Autodesk Inventor part; units mm, degrees
ref_plane "Płaszczyzna konstrukcyjna4" through (813.3596, 0, 43.2274) normal (0.1218693, 0, -0.9925462) x (0, 1, 0)
ref_plane "YZ Plane" through (0, 0, 0) normal (1, 0, 0) x (0, 1, 0)
ref_plane "XZ Plane" through (0, 0, 0) normal (0, 1, 0) x (-1, 0, 0)
sketch "Szkic1" plane through (0, 0, 0) normal (1, 0, 0) x (0, 1, 0)
  circle A0 centre (0, 0) radius 16
  dimension "d0" = 32
extrude "Wyciągnięcie proste1" add sketch "Szkic1" along normal blind 815
shell "Skorupa1" thickness 2 removed faces 2 at (815, 4.7224, 2.4785) at (0, 4.7224, 2.4785)
sketch "Szkic4" plane through (0, 0, 0) normal (0, 0, 1) x (1, 0, 0)
  line L0 (320, 29.1092) -> (320, -35.5658)
  line L1 (0, 16) -> (0, -16)
  point P0 (0, 0)
  dimension "d8" = 320
bend part "Gięcie części1" radius 163.7022 angle 7 line through (320, 29.1092, 0) along (0, -1, 0) centre toward (0, 0, 1) moving side (1, 0, 0) both sides no
sketch "Szkic7" plane through (811.4097, 0, 59.1081) normal (0.9925462, 0, 0.1218693) x (0.1218693, 0, -0.9925462)
  circle A0 centre (0, 0) radius 14
  circle A1 centre (0, 0) radius 16
  point P0 (-40.2184, 0)
  point P1 (16, 0)
ref_plane "Płaszczyzna konstrukcyjna4" through (813.3596, 0, 43.2274) normal (0.1218693, 0, -0.9925462) x (0, 1, 0)
sketch "Szkic8" plane through (813.3596, 0, 43.2274) normal (0.1218693, 0, -0.9925462) x (0, 1, 0)
  line L0 (-19.5179, -302.5651) -> (38.9, -302.5651)
  ellipse E0 centre (0, -812.5651) end of major axis (-16, -812.5651) minor radius 1.9499
  dimension "d15" = 510
bend part "Gięcie części2" radius 35.4407 angle 97 line through (513.0498, -19.5179, 6.354) along (0, 1, 0) centre toward (0.1218693, 0, -0.9925462) moving side (0.9925462, 0, 0.1218693) both sides no
sketch "Szkic10" plane through (0, 0, 0) normal (0, 0, 1) x (1, 0, 0)
  line L0 (0, 16) -> (0, -16) construction
  line L1 (0, -16) -> (320, -16) construction
  line L2 (0, 16) -> (0, -16)
  line L3 (0, -16) -> (2.7996, -16)
  line L4 (2.7996, -16) -> (0, 16)
  point P0 (0, 0)
  dimension "d22" = 5
extrude "Wyciągnięcie proste4" cut sketch "Szkic10" along normal mid plane 32
equation "\"PromieńGięcia\" = Grubość"
equation "\"SzerokośćGięciaPodcięcia\" = Grubość"
equation "\"GłębokośćGięciaPodcięcia\" = 0.5 * Grubość"
equation "\"RozmiarPodcięciaNarożnika\" = 4 * Grubość"
equation "\"MinimalnaPozostałość\" = 2 * Grubość"
equation "\"PromieńPrzejścia\" = PromieńGięcia"
equation "\"Rozmiar_promienia_Jacobiego\" = Grubość"
equation "\"Wielk_odstępu\" = Grubość"
properties part number "Rura_podłużna_ergosiedziska_lewa" material "Aluminium AW-7020"
CAD build for the part. Positions are in the model's coordinates, mm. A direction names the side the tool comes from. Coordinates: 2 decimals unless noted, no trailing zeros. Write each loop counter-clockwise with the first axis right and the second up, starting at its lowest first coordinate (ties: lowest second). Pieces come first, ordered by that corner, then holes.
(1) Two-plate mould, pull along Y, no slides. Class faces 4 (the face through (554.7, 1.1, -271.388)), 5 (the face through (157.848, 12.932, 5.362)), 6 (the face through (423.58, 14.78, 17.66)): +Y half, -Y half, draft (parallel to the pull), parting line (faces both ways), or undercut.
(2) 3-axis set-ups, long thin cutter, end or side, ignore diameter. For faces 1 (the face through (157.76, -3.47, 15.62)), 2 (the face through (584.43, -3.47, -148.41)), 3 (the face through (424.84, 13.354, 7.406)): which of +Z, -Z, +X, -X, +Y, -Y reach the whole face in a straight line?
(3) Cut at A-A, the plane y = 0. List the corners of the cut face in (x, z), and give its area (3 significant figures).
(4) Flat gauge pins, fed straight in: pin 1 (12 mm diameter, centred on y = 1.5, z = -57, fed in from +X); pin 2 (6 mm diameter, centred on x = 242, y = 3, fed in from +Z); pin 3 (1.5 mm diameter, centred on x = 191, y = -3.5, fed in from +Z); pin 4 (10 mm diameter, centred on y = 12.5, z = -104, fed in from +X). Where does each tip first touch, or does it go through?
(5) Cut at B-B, the plane x = 118.5. List the corners of the cut face in (y, z).
(6) Cut at C-C, the plane z = -43. List the corners of the cut face in (x, y), and give its area (3 significant figures).
(7) Drill centre lines: probe 1 along Y at (x, z) = (213.5, 0); probe 2 along X at (y, z) = (0, -104). Where is each one in solid material? Low to high.
Geometry says:
1. face 4: draft
1. face 5: undercut
1. face 6: parting line
2. face 1: -X
2. face 2: -Z
2. face 3: none
3. outline: (1.4, -16) - (320, -16) arc R179.7 ccw to (341.9, -14.66) - (513.05, 6.35) arc R35.44 cw to (552.81, -28.82) - (552.81, -271.39) - (554.81, -271.39) - (554.81, -28.82) arc R37.44 ccw to (512.81, 8.34) - (341.66, -12.68) arc R177.7 cw to (320, -14) - (1.4, -14) - close; (1.4, 14) - (320, 14) arc R149.7 ccw to (338.24, 15.12) - (509.39, 36.13) arc R65.44 cw to (582.81, -28.82) - (582.81, -271.39) - (584.81, -271.39) - (584.81, -28.82) arc R67.44 ccw to (509.15, 38.12) - (338, 17.1) arc R147.7 cw to (320, 16) - (1.4, 16) - close
3. area: 3,360 mm2
4. pin 1: stops at x = 584.81
4. pin 2: stops at z = 16
4. pin 3: stops at z = 15.76
4. pin 4: stops at x = 582.94
5. outline: circle Ø32 at (0, 0); hole circle Ø28 at (0, 0)
6. outline: circle Ø32 at (568.81, 0); hole circle Ø28 at (568.81, 0)
6. area: 188 mm2
7. probe 1: y = -16 to -14, 14 to 16
7. probe 2: x = 552.81 to 554.81, 582.81 to 584.81
